Design review of the part built by this model. Coordinates are the model's own, in mm. A direction names the side the tool comes from. Give positions to 0.01 mm unless a question says otherwise; leave off trailing zeros. Write each loop counter-clockwise with the first axis right and the second up, starting at its lowest first coordinate (ties: lowest second). Pieces come first, ordered by that corner, then holes.
```python
from build123d import *

# Parameters (mm, degrees)
SALIENTE_EXTRUIR3_DEPTH                              = 116
REDONDEO1_R                                          = 5
REDONDEO2_R                                          = 58
REFRENTADO_PARA_TORNILLO_CON_CABEZA_PLAN_D           = 15
REFRENTADO_PARA_TORNILLO_CON_CABEZA_PLAN_CBORE_D     = 30
REFRENTADO_PARA_TORNILLO_CON_CABEZA_PLAN_CBORE_DEPTH = 10
AVELLANADO_PARA_TORNILLO_CON_CABEZA_PLAN_D           = 20
AVELLANADO_PARA_TORNILLO_CON_CABEZA_PLAN_CSINK_D     = 40
AVELLANADO_PARA_TORNILLO_CON_CABEZA_PLAN_CSINK_ANGLE = 75
CORTAR_EXTRUIR1_DEPTH                                = 15


with BuildPart() as part:
    # Croquis1 → Saliente-Extruir3 (new body)
    with BuildSketch(Plane.XY):
        Polygon((0, 164), (0, 228), (-32, 228), (-32, 0), (0, 0), (0, 124), (60, 124), (60, 164), align=None)
    extrude(amount=-SALIENTE_EXTRUIR3_DEPTH)

    # Redondeo1
    redondeo1_edges = [part.edges().sort_by_distance(p)[0] for p in [
        (30, 164, 0),
        (30, 124, 0),
        (30, 164, -116),
        (-16, 228, -116),
        (30, 124, -116),
        (-16, 228, 0),
    ]]
    fillet(redondeo1_edges, radius=REDONDEO1_R)

    # Redondeo2
    redondeo2_edges = [part.edges().sort_by_distance(p)[0] for p in [
        (-16, 0, -116),
        (-16, 0, 0),
    ]]
    fillet(redondeo2_edges, radius=REDONDEO2_R - 0.0001)  # a hair under: the kernel refuses the full size

    # Refrentado para tornillo con cabeza plana de M51 (through all)
    with Locations(Plane(origin=(0, 203, -25), x_dir=(0, 0, 1), z_dir=(1, 0, 0))):
        with Locations((0, 0), (-66, 0)):
            CounterBoreHole(REFRENTADO_PARA_TORNILLO_CON_CABEZA_PLAN_D / 2, REFRENTADO_PARA_TORNILLO_CON_CABEZA_PLAN_CBORE_D / 2, REFRENTADO_PARA_TORNILLO_CON_CABEZA_PLAN_CBORE_DEPTH)

    # Avellanado para tornillo con cabeza plana avellanada de M51 (through all)
    with Locations(Plane(origin=(0, 58, -58), x_dir=(0, 0, 1), z_dir=(1, 0, 0))):
        with Locations((0, 0)):
            CounterSinkHole(AVELLANADO_PARA_TORNILLO_CON_CABEZA_PLAN_D / 2, AVELLANADO_PARA_TORNILLO_CON_CABEZA_PLAN_CSINK_D / 2, counter_sink_angle=AVELLANADO_PARA_TORNILLO_CON_CABEZA_PLAN_CSINK_ANGLE)

    # Croquis6 → Taladro1 (revolve, cut)
    with BuildSketch(Plane(origin=(0, 14, -58), x_dir=(0, 0, -1), z_dir=(0, 1, 0))):
        Polygon((0, 0), (0, 27.819352237), (6, 20), (6, 6.905594024), (12.5, 3), (12.5, 0), align=None)
    revolve(axis=Axis((6.130023899, 14, -58), (-1, 0, 0)), mode=Mode.SUBTRACT)

    # Croquis9 → Taladro2 (revolve, cut)
    with BuildSketch(Plane(origin=(30, 164, -58), x_dir=(0, 0, 1), z_dir=(1, 0, 0))):
        Polygon((0, 0), (0, 40), (10, 40), (20, 0), align=None)
    revolve(axis=Axis((30, 54, -58), (0, 1, 0)), mode=Mode.SUBTRACT)

    # Croquis10 → Cortar-Extruir1 (cut, symmetric)
    with BuildSketch(Plane.XY.offset(-58)):
        Polygon((-32, 228), (0, 228), (0, 213), align=None)
    extrude(amount=CORTAR_EXTRUIR1_DEPTH, both=True, mode=Mode.SUBTRACT)


solid = part.part
```
(1) To check wall thickness, follow L1, parallel to Z at x = -19, y = 203; L2, parallel to Z at x = -2.5, y = 203; L3, parallel to Y at x = -22.5, z = -58. State the ranges of each line that lie inside material, in increasing order.
Resolved:
L1: z = -116 to -98.5, -83.5 to -32.5, -17.5 to 0
L2: z = -116 to -106, -76 to -40, -10 to 0
L3: y = 0 to 9.92, 18.08 to 48, 68 to 223.55
(2) Consider section C-C, the plane z = -96. Give the boundary of the cut face in (x, y), then the cut area to 3 significant figures.
Resolved:
outline: (-32, 14.18) - (0, 14.18) - (0, 124) - (60, 124) - (60, 164) - (0, 164) - (0, 188.86) - (-10, 188.86) - (-10, 197.41) - (-32, 197.41) - close; (-32, 208.59) - (-10, 208.59) - (-10, 217.14) - (0, 217.14) - (0, 228) - (-32, 228) - close
area: 8,710 mm2
(3) Clearance check with flat-ended pins moving along their axes: P1, Ø10, axis at x = 31, z = -50, coming from the -Y side; P2, Ø24, axis at y = 203, z = -25, coming from the +X side; P3, Ø23, axis at y = 58, z = -58, coming from the +X side; P4, Ø12, axis at y = 203, z = -91, coming from the +X side. State where each tip first meets the part, or that it passes through.
Resolved:
P1: stops at y = 124
P2: stops at x = -10
P3: stops at x = -11.08
P4: passes through
(4) Consider section A-A, the plane y = 203. Give the boundary of the cut face in (x, z), then the cut area to 3 significant figures.
Resolved:
outline: (-32, -116) - (0, -116) - (0, -106) - (-10, -106) - (-10, -98.5) - (-32, -98.5) - close; (-32, -83.5) - (-10, -83.5) - (-10, -76) - (0, -76) - (0, -40) - (-10, -40) - (-10, -32.5) - (-32, -32.5) - close; (-32, -17.5) - (-10, -17.5) - (-10, -10) - (0, -10) - (0, 0) - (-32, 0) - close
area: 2,450 mm2
(5) Consider section D-D, the plane y = 113. Give the boundary of the cut face in (x, z), then the cut area to 3 significant figures.
Resolved:
outline: (-32, -116) - (0, -116) - (0, 0) - (-32, 0) - close
area: 3,710 mm2
(6) Consider section B-B, the plane x = 30. Give the boundary of the cut face in (y, z), then the cut area to 3 significant figures.
Resolved:
outline: (124, -111) arc R5 ccw to (129, -116) - (159, -116) arc R5 ccw to (164, -111) - (164, -78) - (124, -68) - close; (124, -48) - (164, -38) - (164, -5) arc R5 ccw to (159, 0) - (129, 0) arc R5 ccw to (124, -5) - close
area: 3,420 mm2
(7) Mouldability with a two-part tool opening along Z and no side actions: class faces 6 (the face through (-32, 116, -57)), 7 (the face through (-23, 58, -48)), 8 (the face through (30, 163, -2)) as pulls with the +Z half, pulls with the -Z half, needs draft (parallel to the pull), parting line crosses it, or undercut.
Resolved:
face 6: needs draft
face 7: undercut
face 8: pulls with the +Z half
(8) Tool access review of faces 1 (the face through (30, 124, -69)), 2 (the face through (30, 125, -2)), 3 (the face through (-12, 222, -43)), 4 (the face through (-16, 227, -2)), 5 (the face through (-1.479, 21.606, -48.08)): name each direction out of +Z, -Z, +X, -X, +Y, -Y from which nothing blocks a thin tool from reaching the whole face with its end or side.
Resolved:
face 1: +Z, -Z, +X, -Y
face 2: +Z, +X, -Y
face 3: +X, +Y
face 4: +Z, +X, -X, +Y
face 5: +X
